Check sheet for the modelled part. Datum: model origin and axes. Units: mm. Face numbers are marked on the shaded views. A direction names the side the tool comes from. Coordinates: 2 decimals unless noted, no trailing zeros. Loops run counter-clockwise (first coordinate to the right, second up) from the corner with the lowest first, then second, coordinate; pieces in that order, holes last. Notation, with made-up numbers: M 49,-33.75 L 61,-33.75 A27 cw 61,4.25 Z; hole C -12.75,63 d10. An arc over 180 degrees is marked long. Write each question's results on one line, items separated by ' | '. Start each with the question number.
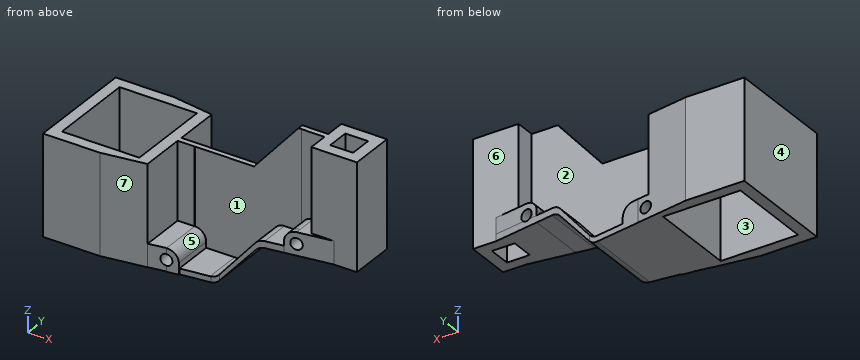
from build123d import *

# Parameters (mm, degrees)
ESQUISSE1_W                   = 68
ESQUISSE1_H                   = 76.5
BOSS_EXTRU_1_DEPTH            = 88
BOSS_EXTRU_4_DEPTH            = 88
ESQUISSE3_W                   = 19.543482411
ESQUISSE3_H                   = 40.235962567
ESQUISSE3_W_2                 = 20.972353068
ESQUISSE3_H_2                 = 40.009358289
ENL_V_MAT_EXTRU_1_DEPTH       = 68
ESQUISSE8_W                   = 10
ESQUISSE8_H                   = 20
BOSS_EXTRU_9_DEPTH            = 96.5
ENL_V_MAT_EXTRU_2_DEPTH       = 140.000518873
ESQUISSE10_R                  = 5
ENL_V_MAT_EXTRU_3_DEPTH       = 170.968886377
ESQUISSE17_W                  = 10
ESQUISSE17_H                  = 4.881451094
BOSS_EXTRU_16_DEPTH           = 68
CONG_2_R                      = 10
BOSS_EXTRU_19_DEPTH           = 56
BOSS_EXTRU_19_DEPTH_BACK      = 85
ESQUISSE19_W                  = 40
ESQUISSE19_H                  = 40
ESQUISSE19_W_2                = 20
ESQUISSE19_H_2                = 20
ESQUISSE20_W                  = 60
ESQUISSE20_H                  = 40
ENL_V_MAT_EXTRU_4_DEPTH       = 216.978999532
ESQUISSE21_W                  = 40
ESQUISSE21_H                  = 10.5
ENL_V_MAT_EXTRU_5_DEPTH       = 216.978999532
ESQUISSE22_W                  = 10
ESQUISSE22_H                  = 20
BOSS_EXTRU_23_DEPTH           = 40
ESQUISSE23_W                  = 10
ESQUISSE23_H                  = 5
BOSS_EXTRU_24_DEPTH           = 93.5
ESQUISSE24_W                  = 10
ESQUISSE24_H                  = 20
BOSS_EXTRU_25_DEPTH           = 40
ESQUISSE25_W                  = 10
ESQUISSE25_H                  = 5
BOSS_EXTRU_26_DEPTH           = 83.5
ESQUISSE26_W                  = 10
ESQUISSE26_H                  = 10
ENL_V_MAT_EXTRU_6_DEPTH       = 211.762136635
CONG_3_R                      = 10
CONG_4_R                      = 10
BOSS_EXTRU_30_DEPTH           = 18
BOSS_EXTRU_30_DEPTH_BACK      = 59
ENL_V_MAT_EXTRU_9_DEPTH       = 180.786479578
BOSS_EXTRU_33_DEPTH           = 20
CONG_8_R                      = 10
ENL_V_MAT_EXTRU_12_DEPTH      = 32
ENL_V_MAT_EXTRU_12_DEPTH_BACK = 210.124791067
ESQUISSE41_R                  = 5
BOSS_EXTRU_34_DEPTH           = 14
BOSS_EXTRU_34_DEPTH_BACK      = 55
ENL_V_MAT_EXTRU_15_DEPTH      = 177.740426159
BOSS_EXTRU_36_REACH           = 178.988
ESQUISSE47_W                  = 84
ESQUISSE47_H                  = 4.881451094
ESQUISSE50_W                  = 75.146765922
ESQUISSE50_H                  = 4.881451094
BOSS_EXTRU_38_DEPTH           = 45.5
ENL_V_MAT_EXTRU_16_DEPTH      = 220.971283896


with BuildPart() as part:
    # Esquisse1 → Boss.-Extru.1 (new body)
    with BuildSketch(Plane.XY):
        Polygon((-111.216373557, -48.25), (-61.216373557, -48.25), (-23.216373557, -42.509358289), (-23.216373557, 42.509358289), (-61.216373557, 48.25), (-111.216373557, 48.25), align=None)
        with Locations((-67.216373557, 0)):
            Rectangle(ESQUISSE1_W, ESQUISSE1_H, mode=Mode.SUBTRACT)
    extrude(amount=BOSS_EXTRU_1_DEPTH)

    # Esquisse2 → Boss.-Extru.4 (add)
    with BuildSketch(Plane.XY.offset(88)):
        Polygon((-8.216373557, 40.469919786), (-59.716373557, 48.25), (-61.216373557, 48.25), (-23.216373557, 42.509358289), (-23.216373557, -42.27382473), (-8.216373557, -39.817862291), align=None)
    extrude(amount=-BOSS_EXTRU_4_DEPTH)

    # Esquisse3 → Enlèv. mat.-Extru.1 (cut)
    with BuildSketch(Plane.XY.offset(88)):
        with Locations((-13.444632352, 22.617981284)):
            Rectangle(ESQUISSE3_W, ESQUISSE3_H)
        with Locations((-12.730197023, -22.504679145)):
            Rectangle(ESQUISSE3_W_2, ESQUISSE3_H_2)
    extrude(amount=-ENL_V_MAT_EXTRU_1_DEPTH, mode=Mode.SUBTRACT)

    # Esquisse8 → Boss.-Extru.9 (add, through all)
    with BuildSketch(Plane.XZ.offset(48.25)):
        with Locations((-3.216373557, 10)):
            Rectangle(ESQUISSE8_W, ESQUISSE8_H)
    extrude(amount=-BOSS_EXTRU_9_DEPTH)

    # Esquisse9 → Enlèv. mat.-Extru.2 (cut, through all)
    with BuildSketch(Plane.XY.offset(20)):
        Polygon((-8.216373557, 48.25), (-8.216373557, 40.469919786), (1.783626443, 38.959224599), (1.783626443, 48.25), align=None)
        Polygon((1.783626443, -48.25), (1.783626443, -38.732620321), (-8.216373557, -40.243315508), (-8.216373557, -48.25), align=None)
    extrude(amount=-ENL_V_MAT_EXTRU_2_DEPTH, mode=Mode.SUBTRACT)

    # Esquisse10 → Enlèv. mat.-Extru.3 (cut, through all)
    with BuildSketch(Plane(origin=(5.760556808, -38.131827365, 0), x_dir=(-0.9887806747234926, -0.149374620646731, 0), z_dir=(0.14937462064673096, -0.9887806747234925, 0))):
        with Locations(Location((14.135521377, -10, 0), (0, 0, 180))):
            Circle(ESQUISSE10_R)
    extrude(amount=-ENL_V_MAT_EXTRU_3_DEPTH, mode=Mode.SUBTRACT)

    # Esquisse17 → Boss.-Extru.16 (add, through all)
    with BuildSketch(Plane.XY.offset(20)):
        with Locations((-3.216373557, 0.059274453)):
            Rectangle(ESQUISSE17_W, ESQUISSE17_H)
    extrude(amount=BOSS_EXTRU_16_DEPTH)

    # Congé2
    cong_2_edges = [part.edges().sort_by_distance(p)[0] for p in [
        (1.783626443, 20.729612299, 20),
        (1.783626443, -20.557035707, 20),
    ]]
    fillet(cong_2_edges, radius=CONG_2_R - 0.0001)  # a hair under: the kernel refuses the full size

    # Esquisse34 → Boss.-Extru.30 (add, two sides: drawn at the far end of the back side and taken through both)
    with BuildSketch(Plane.XZ.offset(20).offset(-BOSS_EXTRU_30_DEPTH_BACK)):
        with BuildLine():
            Line((34.377909415, 8.572123903), (34.370735232, 3.444656645))
            ThreePointArc((34.370735232, 3.444656645), (30.969175902, 0.901828933), (26.819081539, 0))
            Line((26.819081539, 0), (1.783626443, 0))
            Line((1.783626443, 0), (1.783626443, 5))
            Line((1.783626443, 5), (26.717464984, 5))
            ThreePointArc((26.717464984, 5), (30.943647601, 5.93692213), (34.377909415, 8.572123903))
        make_face()
    extrude(amount=BOSS_EXTRU_30_DEPTH + BOSS_EXTRU_30_DEPTH_BACK)

    # Esquisse35 → Enlèv. mat.-Extru.9 (cut, through all)
    with BuildSketch(Plane(origin=(0, 0, 40), x_dir=(-1, 0, 0), z_dir=(0, 0, -1))):
        Polygon((0, -39.002071909), (-46.91486771, -31.914665424), (-9.768949851, -63.05793836), align=None)
        Polygon((-56.81735982, 58.483787391), (-46.91486771, 32.011010427), (13.201496413, 41.166197955), (13.201496413, 63.711388499), align=None)
    extrude(amount=ENL_V_MAT_EXTRU_9_DEPTH, mode=Mode.SUBTRACT)



with BuildPart() as body_2:
    # Esquisse19 → Boss.-Extru.19 (new, two sides: drawn at the far end of the back side and taken through both)
    with BuildSketch(Plane.XY.offset(88).offset(-BOSS_EXTRU_19_DEPTH_BACK)):
        with Locations((125.783626443, 0)):
            Rectangle(ESQUISSE19_W, ESQUISSE19_H)
        with Locations((125.783626443, 0)):
            Rectangle(ESQUISSE19_W_2, ESQUISSE19_H_2, mode=Mode.SUBTRACT)
    extrude(amount=BOSS_EXTRU_19_DEPTH + BOSS_EXTRU_19_DEPTH_BACK)

    # Esquisse20 → Enlèv. mat.-Extru.4 (cut, through all)
    with BuildSketch(Plane.XZ.offset(20)):
        with Locations((134.192494857, 20)):
            Rectangle(ESQUISSE20_W, ESQUISSE20_H)
    extrude(amount=-ENL_V_MAT_EXTRU_4_DEPTH, mode=Mode.SUBTRACT)

    # Esquisse21 → Enlèv. mat.-Extru.5 (cut, through all)
    with BuildSketch(Plane.XZ.offset(20)):
        with Locations((125.783626443, 138.75)):
            Rectangle(ESQUISSE21_W, ESQUISSE21_H)
    extrude(amount=-ENL_V_MAT_EXTRU_5_DEPTH, mode=Mode.SUBTRACT)

    # Esquisse22 → Boss.-Extru.23 (add)
    with BuildSketch(Plane.XZ.offset(20)):
        with Locations((100.783626443, 50)):
            Rectangle(ESQUISSE22_W, ESQUISSE22_H)
    extrude(amount=-BOSS_EXTRU_23_DEPTH)

    # Esquisse23 → Boss.-Extru.24 (add)
    with BuildSketch(Plane.XY.offset(133.5)):
        with Locations((100.783626443, 0)):
            Rectangle(ESQUISSE23_W, ESQUISSE23_H)
    extrude(amount=-BOSS_EXTRU_24_DEPTH)

    # Esquisse24 → Boss.-Extru.25 (add)
    with BuildSketch(Plane.XZ.offset(20)):
        with Locations((90.783626443, 50)):
            Rectangle(ESQUISSE24_W, ESQUISSE24_H)
    extrude(amount=-BOSS_EXTRU_25_DEPTH)

    # Esquisse25 → Boss.-Extru.26 (add)
    with BuildSketch(Plane.XY.offset(60)):
        with Locations((90.783626443, 0)):
            Rectangle(ESQUISSE25_W, ESQUISSE25_H)
    extrude(amount=BOSS_EXTRU_26_DEPTH)

    # Esquisse26 → Enlèv. mat.-Extru.6 (cut, through all)
    with BuildSketch(Plane.XZ.offset(2.5)):
        with Locations((90.783626443, 138.5)):
            Rectangle(ESQUISSE26_W, ESQUISSE26_H)
    extrude(amount=-ENL_V_MAT_EXTRU_6_DEPTH, mode=Mode.SUBTRACT)

    # Congé3
    cong_3_edges = [body_2.edges().sort_by_distance(p)[0] for p in [
        (85.783626443, -11.25, 60),
    ]]
    fillet(cong_3_edges, radius=CONG_3_R)

    # Congé4
    cong_4_edges = [body_2.edges().sort_by_distance(p)[0] for p in [
        (85.783626443, 11.25, 60),
    ]]
    fillet(cong_4_edges, radius=CONG_4_R)

    # Esquisse40 → Boss.-Extru.33 (add)
    with BuildSketch(Plane(origin=(0, 0, 40), x_dir=(-1, 0, 0), z_dir=(0, 0, -1))):
        Polygon((-85.783626443, -20), (-125.783626443, -20), (-85.783626443, -26.042780749), align=None)
        Polygon((-85.783626443, 26.105828189), (-125.783626443, 20), (-85.783626443, 20), align=None)
    extrude(amount=-BOSS_EXTRU_33_DEPTH)

    # Congé8
    cong_8_edges = [body_2.edges().sort_by_distance(p)[0] for p in [
        (85.783626443, -23.021390374, 60),
        (85.783626443, 23.052914094, 60),
    ]]
    fillet(cong_8_edges, radius=CONG_8_R)

    # Esquisse41 → Enlèv. mat.-Extru.12 (cut, two sides: drawn at the far end of the back side and taken through both)
    with BuildSketch(Plane.XZ.offset(20).offset(-ENL_V_MAT_EXTRU_12_DEPTH_BACK)):
        with Locations(Location((95.783626443, 50, 0), (0, 0, 180))):
            Circle(ESQUISSE41_R)
    extrude(amount=ENL_V_MAT_EXTRU_12_DEPTH + ENL_V_MAT_EXTRU_12_DEPTH_BACK, mode=Mode.SUBTRACT)


with BuildPart() as part_1:
    add(part.part)

    add(body_2.part)  # Boss.-Extru.34 merges body 2
    # Esquisse42 → Boss.-Extru.34 (add, two sides: drawn at the far end of the back side and taken through both)
    with BuildSketch(Plane.XZ.offset(20).offset(-BOSS_EXTRU_34_DEPTH_BACK)):
        with BuildLine():
            Line((85.783626443, 46), (70.446703025, 46))
            ThreePointArc((70.446703025, 46), (66.220520407, 45.06307787), (62.786258594, 42.427876097))
            Line((62.786258594, 42.427876097), (34.377909415, 8.572123903))
            Line((34.377909415, 8.572123903), (34.370735232, 3.444656645))
            Line((34.370735232, 3.444656645), (63.202936222, 36.658904216))
            ThreePointArc((63.202936222, 36.658904216), (66.635938394, 39.216008921), (70.823654148, 40.103322365))
            Line((70.823654148, 40.103322365), (85.783626443, 40))
            Line((85.783626443, 40), (85.783626443, 46))
        make_face()
    extrude(amount=BOSS_EXTRU_34_DEPTH + BOSS_EXTRU_34_DEPTH_BACK)

    # Esquisse46 → Enlèv. mat.-Extru.15 (cut, through all)
    with BuildSketch(Plane.XY.offset(46)):
        Polygon((125.783626443, 20), (1.783626443, 38.884097035), (91.450217157, 42.474258999), align=None)
        Polygon((125.783626443, -20), (34.377909415, -34), (1.783626443, -38), (94.864318468, -42.795104314), align=None)
    extrude(amount=-ENL_V_MAT_EXTRU_15_DEPTH, mode=Mode.SUBTRACT)

    # Esquisse47 → Boss.-Extru.36 (add, up to next)
    with BuildSketch(Plane.XY.offset(88), mode=Mode.PRIVATE) as boss_extru_36_sk1:
        with Locations((43.783626443, 0.059274453)):
            Rectangle(ESQUISSE47_W, ESQUISSE47_H)
    boss_extru_36_tool1 = extrude(boss_extru_36_sk1.sketch, amount=-BOSS_EXTRU_36_REACH, mode=Mode.PRIVATE) - part_1.part
    add(boss_extru_36_tool1.solids().sort_by_distance((43.783626, 0.059274, 88))[0])

    # Esquisse50 → Boss.-Extru.38 (add, through all)
    with BuildSketch(Plane.XY.offset(88)):
        with Locations((48.32250802, 0.059274453)):
            Rectangle(ESQUISSE50_W, ESQUISSE50_H)
    extrude(amount=BOSS_EXTRU_38_DEPTH)

    # Esquisse51 → Enlèv. mat.-Extru.16 (cut, through all)
    with BuildSketch(Plane.XZ.offset(48.25)):
        Polygon((82.955365358, 133.5), (10.749125059, 133.5), (10.749125059, 88), (43.801721697, 88), align=None)
    extrude(amount=-ENL_V_MAT_EXTRU_16_DEPTH, mode=Mode.SUBTRACT)


solid = part_1.part
1) Gauge pin test, flat ends, axial feed: P1, Ø1, axis at x = 59.5, z = 103.5, coming from the +Y side; P2, Ø12, axis at x = -14.5, y = -22, coming from the +Z side; P3, Ø3, axis at x = 92, z = 55.5, coming from the -Y side. Record the tip position at first contact, or that the pin passes through.
2) Section check D-D (z = 118.5). Enter the section's corners in (x, y).
3) Section check B-B (z = 68). Enter the section's corners in (x, y).
4) Release check for a two-part mould opening along X. For the marked faces 4, 5, 6 and 7 record: +X half, -X half, draft (parallel to the pull), parting line (faces both ways), or undercut.
5) Set-up check for the marked faces 1, 2 and 3: record each of +Z, -Z, +X, -X, +Y, -Y from which the full face is reachable in a straight line by a thin tool's end or side.
6) Thickness scan on probe 1 along X at (y, z) = (12, 50); probe 2 along X at (y, z) = (3, 50); probe 3 along X at (y, z) = (-0.5, 50). Record the ranges inside material, lowest first.
7) Section check C-C (z = 92). Enter the section's corners in (x, y), then the cut area to 3 significant figures.
8) Section check A-A (x = -79). Enter the section's corners in (y, z), then the cut area to 3 significant figures.
Return value:
1) P1: stops at y = 2.5 | P2: stops at z = 20 | P3: stops at y = -25.33
2) outline: M 70.05,-2.38 L 85.78,-2.38 L 85.78,-2.5 L 105.78,-2.5 L 105.78,-20 L 145.78,-20 L 145.78,20 L 105.78,20 L 105.78,2.5 L 70.05,2.5 Z; hole M 115.78,-10 L 135.78,-10 L 135.78,10 L 115.78,10 Z
3) outline: M -111.22,-48.25 L -61.22,-48.25 L -23.22,-42.51 L -23.22,-2.5 L -8.22,-2.5 L -8.22,-2.38 L 85.78,-2.38 L 85.78,-2.5 L 105.78,-2.5 L 105.78,-20 L 145.78,-20 L 145.78,20 L 105.78,20 L 105.78,2.5 L -23.22,2.5 L -23.22,42.74 L -59.72,48.25 L -111.22,48.25 Z; hole M -101.22,-38.25 L -33.22,-38.25 L -33.22,38.25 L -101.22,38.25 Z; hole M 115.78,-10 L 135.78,-10 L 135.78,10 L 115.78,10 Z
4) face 4: -X half | face 5: undercut | face 6: draft | face 7: +X half
5) face 1: +Z, -Y | face 2: +Z, +Y | face 3: +Z, -Z
6) probe 1: x = -111.22 to -101.22, -33.22 to -23.22, 85.78 to 90.78, 100.78 to 145.78 | probe 2: x = -111.22 to -101.22, -33.22 to -23.22, 85.78 to 90.78, 100.78 to 115.78, 135.78 to 145.78 | probe 3: x = -111.22 to -101.22, -33.22 to 90.78, 100.78 to 115.78, 135.78 to 145.78
7) outline: M 47.24,-2.38 L 85.78,-2.38 L 85.78,-2.5 L 105.78,-2.5 L 105.78,-20 L 145.78,-20 L 145.78,20 L 105.78,20 L 105.78,2.5 L 47.24,2.5 Z; hole M 115.78,-10 L 135.78,-10 L 135.78,10 L 115.78,10 Z | area: 1,490 mm2
8) outline: M -48.25,0 L -38.25,0 L -38.25,88 L -48.25,88 Z; M 38.25,0 L 48.25,0 L 48.25,88 L 38.25,88 Z | area: 1,760 mm2
